from build123d import *

# Parameters (mm, degrees)
BOSS_EXTRUDE1_DEPTH = 33
SKETCH2_W           = 50
SKETCH2_H           = 15
BOSS_EXTRUDE2_DEPTH = 400


with BuildPart() as part:
    # Sketch1 → Boss-Extrude1 (new body)
    with BuildSketch(Plane.XY):
        with BuildLine():
            Line((0, 0), (0, -480))
            Line((0, -480), (-625, -480))
            Line((-625, -480), (-625, -80))
            Line((-625, -80), (-525, -80))
            add(Edge.make_bspline(
                [(0, 0), (-83.701492577, 2.102656983), (-263.298331294, -12.316995698), (-428.0447482, -87.215369033), (-525, -80)],
                knots=[0, 0, 0, 0, 0.472195636, 1, 1, 1, 1], degree=3))
        make_face()
    boss_extrude1 = extrude(amount=BOSS_EXTRUDE1_DEPTH)

    # Sketch2 → Boss-Extrude2 (add, through all)
    with BuildSketch(Plane(origin=(0, -80, 0), x_dir=(1, 0, 0), z_dir=(0, 1, 0))):
        with Locations((-650, -16.5)):
            Rectangle(SKETCH2_W, SKETCH2_H)
    boss_extrude2 = extrude(amount=-BOSS_EXTRUDE2_DEPTH)

    # Mirror2: Boss-Extrude1, Boss-Extrude2 across plane
    add(boss_extrude1.mirror(Plane(origin=(0, 0, 0), x_dir=(0, 0, 1), z_dir=(1, 0, 0))))
    add(boss_extrude2.mirror(Plane(origin=(0, 0, 0), x_dir=(0, 0, 1), z_dir=(1, 0, 0))))


solid = part.part
Geometry check sheet. Reference: the model listing, model coordinates, mm. A direction names the side the tool comes from. Give positions to 0.01 mm unless a question says otherwise; leave off trailing zeros. Loops run counter-clockwise (first coordinate to the right, second up) from the corner with the lowest first, then second, coordinate; pieces in that order, holes last. Notation, with made-up numbers: (30, 12) -> (88, 12) arc R18 cw to (88, 25) -> close; hole circle Ø8 at (-23, 61). An arc over 180 degrees is marked (long way). Answer in a Markdown table with one row per item. Add a question column.
1) Gauge pin test, flat ends, axial feed: P1, Ø10, axis at y = -285, z = 29.5, coming from the -X side; P2, Ø2.5, axis at y = -261.5, z = 5, coming from the +X side; P3, Ø15, axis at x = 649, y = -290, coming from the +Z side. Record the tip position at first contact, or that the pin passes through.
2) Material ranges on probe 1 along Y at (x, z) = (-572, 9); probe 2 along X at (y, z) = (-242, 8); probe 3 along Y at (x, z) = (156, 20.5), recorded low to high. Write a range as from..to.
3) Set-up check for faces 1 (the face through (-584, -80, 16)), 2 (the face through (650, -277, 9)), 3 (the face through (584, -80, 16)), 4 (the face through (-650, -277, 9)): record each of +Z, -Z, +X, -X, +Y, -Y from which the full face is reachable in a straight line by a thin tool's end or side.
4) Cross-section at A-A on y = -188. Record the boundary of the cut face in (x, z), and give its area (4 significant figures).
Outcome:
| question | item | result |
|---|---|---|
| 1 | P1 | stops at x = -625 |
| 1 | P2 | stops at x = 625 |
| 1 | P3 | stops at z = 24 |
| 2 | probe 1 | y = -480..-80 |
| 2 | probe 2 | x = -625..625 |
| 2 | probe 3 | y = -480..-7.47 |
| 3 | face 1 | +Z, -Z, -X, +Y |
| 3 | face 2 | -Z, +X, +Y, -Y |
| 3 | face 3 | +Z, -Z, +X, +Y |
| 3 | face 4 | -Z, -X, +Y, -Y |
| 4 | outline | (-675, 9) -> (-625, 9) -> (-625, 0) -> (625, 0) -> (625, 9) -> (675, 9) -> (675, 24) -> (625, 24) -> (625, 33) -> (-625, 33) -> (-625, 24) -> (-675, 24) -> close |
| 4 | area | 42,750 mm^2 |
